Build history of the part. All positions in model axes, mm. Coordinates: 2 decimals unless noted, no trailing zeros. Write each loop counter-clockwise with the first axis right and the second up, starting at its lowest first coordinate (ties: lowest second). Pieces come first, ordered by that corner, then holes.
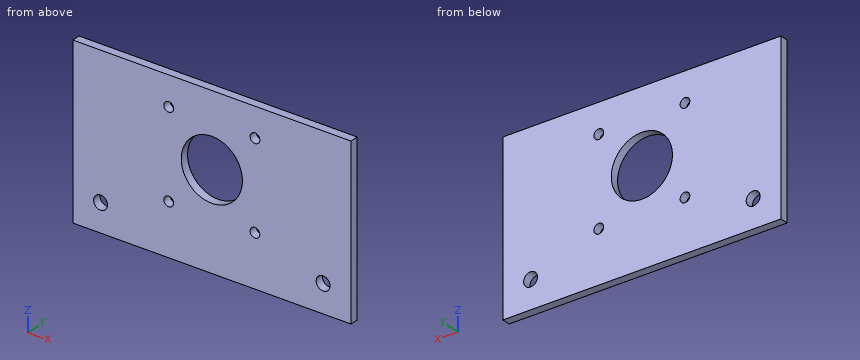
from build123d import *

# Parameters (mm, degrees)
SKETCH1_W          = 100
SKETCH1_H          = 60
BASE_FLANGE1_DEPTH = 3
SKETCH6_R          = 2.5
SKETCH6_R_2        = 11
SKETCH6_R_3        = 1.75
CUT_EXTRUDE1_DEPTH = 10


# Sheet-metal steps are written as plain solids
with BuildPart() as part:
    # Sketch1 → Base-Flange1 (new body)
    with BuildSketch(Plane(origin=(0, 0, 0), x_dir=(1, 0, 0), z_dir=(0, 1, 0))):
        Rectangle(SKETCH1_W, SKETCH1_H)
    extrude(amount=-BASE_FLANGE1_DEPTH)

    # Sketch6 → Cut-Extrude1 (cut)
    with BuildSketch(Plane(origin=(0, 0, 0), x_dir=(1, 0, 0), z_dir=(0, 1, 0))):
        with Locations(Location((40, 20, 0), (0, 0, 270))):
            Circle(SKETCH6_R)
        with Locations(Location((-40, 20, 0), (0, 0, 90))):
            Circle(SKETCH6_R)
        with Locations(Location((0, -4, 0), (0, 0, 270))):
            Circle(SKETCH6_R_2)
        with Locations(Location((15.5, 11.5, 0), (0, 0, 270))):
            Circle(SKETCH6_R_3)
        with Locations(Location((15.5, -19.5, 0), (0, 0, 90))):
            Circle(SKETCH6_R_3)
        with Locations(Location((-15.5, -19.5, 0), (0, 0, 270))):
            Circle(SKETCH6_R_3)
        with Locations(Location((-15.5, 11.5, 0), (0, 0, 90))):
            Circle(SKETCH6_R_3)
    extrude(amount=-CUT_EXTRUDE1_DEPTH, mode=Mode.SUBTRACT)


solid = part.part
(1) Slice it at D-D, the plane z = 4. List the corners of the cut face in (x, y).
(2) Probe L1, parallel to X at y = -0.9, z = -20; L2, parallel to Z at x = -40, y = -1.7; L3, parallel to Z at x = 17, y = -2.15. List the from-to ranges inside material, lowest first.
(3) Slice it at B-B, the plane z = -18.5. List the corners of the cut face in (x, y), and give its area (3 significant figures).
(4) Slice it at C-C, the plane x = 15.5. List the corners of the cut face in (y, z), and give its area (3 significant figures).
(5) Slice it at A-A, the plane x = 40. List the corners of the cut face in (y, z), and give its area (3 significant figures).
Results:
1. outline: (-50, -3) - (-11, -3) - (-11, 0) - (-50, 0) - close; (11, -3) - (50, -3) - (50, 0) - (11, 0) - close
2. L1: x = -50 to -42.5, -37.5 to 37.5, 42.5 to 50
2. L2: z = -30 to -22.5, -17.5 to 30
2. L3: z = -30 to -12.4, -10.6 to 18.6, 20.4 to 30
3. outline: (-50, -3) - (-42, -3) - (-42, 0) - (-50, 0) - close; (-38, -3) - (38, -3) - (38, 0) - (-38, 0) - close; (42, -3) - (50, -3) - (50, 0) - (42, 0) - close
3. area: 276 mm2
4. outline: (-3, -30) - (0, -30) - (0, -13.25) - (-3, -13.25) - close; (-3, -9.75) - (0, -9.75) - (0, 17.75) - (-3, 17.75) - close; (-3, 21.25) - (0, 21.25) - (0, 30) - (-3, 30) - close
4. area: 159 mm2
5. outline: (-3, -30) - (0, -30) - (0, -22.5) - (-3, -22.5) - close; (-3, -17.5) - (0, -17.5) - (0, 30) - (-3, 30) - close
5. area: 165 mm2
